```python
from build123d import *

# Parameters (mm, degrees)
SKETCH1_W                           = 170
SKETCH1_H                           = 60
SKETCH1_W_2                         = 53
SKETCH1_H_2                         = 30
BOSS_EXTRUDE1_DEPTH                 = 5
SKETCH3_W                           = 40
SKETCH3_H                           = 24
CUT_EXTRUDE1_DEPTH                  = 5
SKETCH5_R                           = 3
CUT_EXTRUDE2_DEPTH                  = 10
SKETCH6_R                           = 3
SKETCH6_R_2                         = 1.375
BOSS_EXTRUDE2_DEPTH                 = 5
SKETCH8_R                           = 2.375
SKETCH8_R_2                         = 1.375
BOSS_EXTRUDE3_DEPTH                 = 10
SKETCH9_W                           = 53
SKETCH9_H                           = 25
SKETCH9_W_2                         = 43
SKETCH9_H_2                         = 17.5
BOSS_EXTRUDE4_DEPTH                 = 5
SKETCH10_W                          = 3
SKETCH10_H                          = 17.5
SKETCH10_W_2                        = 5
SKETCH10_W_3                        = 2
BOSS_EXTRUDE5_DEPTH                 = 2
SKETCH11_W                          = 5
SKETCH11_H                          = 17.5
CUT_EXTRUDE5_DEPTH                  = 2
CHAMFER1_SIZE                       = 5
FILLET1_R                           = 5
SKETCH12_W                          = 43
SKETCH12_H                          = 32.847222222
SKETCH12_W_2                        = 60
SKETCH12_H_2                        = 24.8
CUT_EXTRUDE6_DEPTH                  = 105.522724802
FILLET2_R                           = 5
F_2_8_2_8_DIAMETER_HOLE1_AT_2_COUNT = 2
F_2_8_2_8_DIAMETER_HOLE1_AT_2_PITCH = 53.036757065
F_2_8_2_8_DIAMETER_HOLE1_AT_3_COUNT = 2
F_2_8_2_8_DIAMETER_HOLE1_AT_3_PITCH = 79.966896276
F_2_8_2_8_DIAMETER_HOLE1_AT_4_COUNT = 2
F_2_8_2_8_DIAMETER_HOLE1_AT_4_PITCH = 48.276707634
F_2_8_2_8_DIAMETER_HOLE1_AT_5_COUNT = 2
F_2_8_2_8_DIAMETER_HOLE1_AT_5_PITCH = 66.671976122
F_2_8_2_8_DIAMETER_HOLE1_AT_6_COUNT = 2
F_2_8_2_8_DIAMETER_HOLE1_AT_6_PITCH = 92.923433535
F_2_8_2_8_DIAMETER_HOLE1_AT_7_COUNT = 2
F_2_8_2_8_DIAMETER_HOLE1_AT_7_PITCH = 160.77550964
F_2_8_2_8_DIAMETER_HOLE1_AT_8_COUNT = 2
F_2_8_2_8_DIAMETER_HOLE1_AT_8_PITCH = 153.65124308


with BuildPart() as part:
    # Sketch1 → Boss-Extrude1 (new body)
    with BuildSketch(Plane(origin=(0, 0, 0), x_dir=(1, 0, 0), z_dir=(0, 1, 0))):
        Rectangle(SKETCH1_W, SKETCH1_H)
        with Locations((58.5, 45)):
            Rectangle(SKETCH1_W_2, SKETCH1_H_2)
    extrude(amount=BOSS_EXTRUDE1_DEPTH)

    # Sketch3 → Cut-Extrude1 (cut)
    with BuildSketch(Plane(origin=(0, 5, 0), x_dir=(1, 0, 0), z_dir=(0, 1, 0))):
        with Locations((12, 18)):
            Rectangle(SKETCH3_W, SKETCH3_H)
    extrude(amount=-CUT_EXTRUDE1_DEPTH, mode=Mode.SUBTRACT)

    # Sketch5 → Cut-Extrude2 (cut)
    with BuildSketch(Plane.XZ):
        with Locations(Location((-77.5, 22.5, 0), (0, 0, 270))):
            Circle(SKETCH5_R)
    extrude(amount=-CUT_EXTRUDE2_DEPTH, mode=Mode.SUBTRACT)

    # Sketch6 → Boss-Extrude2 (add)
    # profile 1 of 4: a face of its own
    with BuildSketch(Plane(origin=(0, 5, 0), x_dir=(1, 0, 0), z_dir=(0, 1, 0))):
        with Locations(Location((-71.03, -24.13, 0), (0, 0, 270))):
            Circle(SKETCH6_R)
        with Locations(Location((-71.03, -24.13, 0), (0, 0, 270))):
            Circle(SKETCH6_R_2, mode=Mode.SUBTRACT)
    # profile 2 of 4: a face of its own
    with BuildSketch(Plane(origin=(0, 5, 0), x_dir=(1, 0, 0), z_dir=(0, 1, 0))):
        with Locations(Location((-69.76, 24.13, 0), (0, 0, 270))):
            Circle(SKETCH6_R)
        with Locations(Location((-69.76, 24.13, 0), (0, 0, 270))):
            Circle(SKETCH6_R_2, mode=Mode.SUBTRACT)
    # profile 3 of 4: a face of its own
    with BuildSketch(Plane(origin=(0, 5, 0), x_dir=(1, 0, 0), z_dir=(0, 1, 0))):
        with Locations(Location((-18.96, -19.05, 0), (0, 0, 270))):
            Circle(SKETCH6_R)
        with Locations(Location((-18.96, -19.05, 0), (0, 0, 270))):
            Circle(SKETCH6_R_2, mode=Mode.SUBTRACT)
    # profile 4 of 4: a face of its own
    with BuildSketch(Plane(origin=(0, 5, 0), x_dir=(1, 0, 0), z_dir=(0, 1, 0))):
        with Locations(Location((-18.96, 8.89, 0), (0, 0, 270))):
            Circle(SKETCH6_R)
        with Locations(Location((-18.96, 8.89, 0), (0, 0, 270))):
            Circle(SKETCH6_R_2, mode=Mode.SUBTRACT)
    extrude(amount=BOSS_EXTRUDE2_DEPTH)

    # Sketch8 → Boss-Extrude3 (add)
    # profile 1 of 4: a face of its own
    with BuildSketch(Plane(origin=(0, 5, 0), x_dir=(1, 0, 0), z_dir=(0, 1, 0))):
        with Locations(Location((7.5, 3.5, 0), (0, 0, 270))):
            Circle(SKETCH8_R)
        with Locations(Location((7.5, 3.5, 0), (0, 0, 270))):
            Circle(SKETCH8_R_2, mode=Mode.SUBTRACT)
    # profile 2 of 4: a face of its own
    with BuildSketch(Plane(origin=(0, 5, 0), x_dir=(1, 0, 0), z_dir=(0, 1, 0))):
        with Locations(Location((7.5, -27.5, 0), (0, 0, 270))):
            Circle(SKETCH8_R)
        with Locations(Location((7.5, -27.5, 0), (0, 0, 270))):
            Circle(SKETCH8_R_2, mode=Mode.SUBTRACT)
    # profile 3 of 4: a face of its own
    with BuildSketch(Plane(origin=(0, 5, 0), x_dir=(1, 0, 0), z_dir=(0, 1, 0))):
        with Locations(Location((82.5, -27.5, 0), (0, 0, 270))):
            Circle(SKETCH8_R)
        with Locations(Location((82.5, -27.5, 0), (0, 0, 270))):
            Circle(SKETCH8_R_2, mode=Mode.SUBTRACT)
    # profile 4 of 4: a face of its own
    with BuildSketch(Plane(origin=(0, 5, 0), x_dir=(1, 0, 0), z_dir=(0, 1, 0))):
        with Locations(Location((82.5, 3.5, 0), (0, 0, 270))):
            Circle(SKETCH8_R)
        with Locations(Location((82.5, 3.5, 0), (0, 0, 270))):
            Circle(SKETCH8_R_2, mode=Mode.SUBTRACT)
    extrude(amount=BOSS_EXTRUDE3_DEPTH)

    # Sketch9 → Boss-Extrude4 (add)
    # profile 1 of 2: a face of its own
    with BuildSketch(Plane(origin=(0, 5, 0), x_dir=(1, 0, 0), z_dir=(0, 1, 0))):
        with Locations((58.5, 47.5)):
            Rectangle(SKETCH9_W, SKETCH9_H)
        with Locations((58.5, 46.25)):
            Rectangle(SKETCH9_W_2, SKETCH9_H_2, mode=Mode.SUBTRACT)
    # profile 2 of 2: a face of its own
    with BuildSketch(Plane(origin=(0, 5, 0), x_dir=(1, 0, 0), z_dir=(0, 1, 0))):
        with Locations((58.5, 20)):
            Rectangle(SKETCH9_W, SKETCH9_H)
        with Locations((58.5, 21.25)):
            Rectangle(SKETCH9_W_2, SKETCH9_H_2, mode=Mode.SUBTRACT)
    extrude(amount=BOSS_EXTRUDE4_DEPTH)

    # Sketch10 → Boss-Extrude5 (add)
    with BuildSketch(Plane(origin=(0, 5, 0), x_dir=(1, 0, 0), z_dir=(0, 1, 0))):
        with Locations((45.5, 21.25)):
            Rectangle(SKETCH10_W, SKETCH10_H)
        with Locations((59.5, 21.25)):
            Rectangle(SKETCH10_W_2, SKETCH10_H)
        with Locations((70, 21.25)):
            Rectangle(SKETCH10_W_3, SKETCH10_H)
        with Locations((45.5, 46.25)):
            Rectangle(SKETCH10_W, SKETCH10_H)
        with Locations((59.5, 46.25)):
            Rectangle(SKETCH10_W_2, SKETCH10_H)
        with Locations((70, 46.25)):
            Rectangle(SKETCH10_W_3, SKETCH10_H)
        with Locations((79, 21.25)):
            Rectangle(SKETCH10_W_3, SKETCH10_H)
        with Locations((79, 46.25)):
            Rectangle(SKETCH10_W_3, SKETCH10_H)
    extrude(amount=BOSS_EXTRUDE5_DEPTH)

    # Sketch11 → Cut-Extrude5 (cut)
    with BuildSketch(Plane(origin=(0, 10, 0), x_dir=(1, 0, 0), z_dir=(0, 1, 0))):
        with Locations((82.5, 21.25)):
            Rectangle(SKETCH11_W, SKETCH11_H)
        with Locations((82.5, 46.25)):
            Rectangle(SKETCH11_W, SKETCH11_H)
    extrude(amount=-CUT_EXTRUDE5_DEPTH, mode=Mode.SUBTRACT)

    # Chamfer1
    chamfer1_edges = [part.edges().sort_by_distance(p)[0] for p in [
        (-85, 2.5, 30),
        (-85, 2.5, -30),
        (-8, 2.5, -30),
        (32, 5, -60),
        (85, 5, -60),
    ]]
    chamfer(chamfer1_edges, length=CHAMFER1_SIZE)

    # Fillet1
    fillet1_edges = [part.edges().sort_by_distance(p)[0] for p in [
        (-8, 2.5, -6),
    ]]
    fillet(fillet1_edges, radius=FILLET1_R)

    # Sketch12 → Cut-Extrude6 (cut, through all)
    with BuildSketch(Plane(origin=(0, 5, 0), x_dir=(1, 0, 0), z_dir=(0, 1, 0))):
        with Locations((-46.5, 0)):
            Rectangle(SKETCH12_W, SKETCH12_H)
        with Locations((45, -12)):
            Rectangle(SKETCH12_W_2, SKETCH12_H_2)
    extrude(amount=-CUT_EXTRUDE6_DEPTH, mode=Mode.SUBTRACT)

    # Fillet2
    fillet2_edges = [part.edges().sort_by_distance(p)[0] for p in [
        (-25, 2.5, -16.423611111),
        (-25, 2.5, 16.423611111),
        (-68, 2.5, 16.423611111),
        (-68, 2.5, -16.423611111),
        (75, 2.5, -0.4),
        (75, 2.5, 24.4),
        (15, 2.5, 24.4),
        (15, 2.5, -0.4),
    ]]
    fillet(fillet2_edges, radius=FILLET2_R)

    # Sketch14 → Ø2.8 (2.8) Diameter Hole1 (revolve, cut)
    with BuildSketch(Plane(origin=(-69.76, 5, -24.13), x_dir=(0, 0, 1), z_dir=(1, 0, 0))):
        Polygon((0, 0), (0, 10.841204867), (1.4, 10), (1.4, 0), align=None)
    f_2_8_2_8_diameter_hole1 = revolve(axis=Axis((-69.76, 11.35, -24.13), (0, -1, 0)), mode=Mode.SUBTRACT)

    # Ø2.8 (2.8) Diameter Hole1 at 2: Ø2.8 (2.8) Diameter Hole1 ×2
    with Locations(*[Vector(0.9578262852211514, 0, 0.2873478855663455) * (i * F_2_8_2_8_DIAMETER_HOLE1_AT_2_PITCH) for i in range(1, F_2_8_2_8_DIAMETER_HOLE1_AT_2_COUNT)]):
        add(f_2_8_2_8_diameter_hole1, mode=Mode.SUBTRACT)

    # Ø2.8 (2.8) Diameter Hole1 at 3: Ø2.8 (2.8) Diameter Hole1 ×2
    with Locations(*[Vector(0.9661497894509072, 0, 0.2579817519592574) * (i * F_2_8_2_8_DIAMETER_HOLE1_AT_3_PITCH) for i in range(1, F_2_8_2_8_DIAMETER_HOLE1_AT_3_COUNT)]):
        add(f_2_8_2_8_diameter_hole1, mode=Mode.SUBTRACT)

    # Ø2.8 (2.8) Diameter Hole1 at 4: Ø2.8 (2.8) Diameter Hole1 ×2
    with Locations(*[Vector(-0.02630668208823303, 0, 0.9996539193528472) * (i * F_2_8_2_8_DIAMETER_HOLE1_AT_4_PITCH) for i in range(1, F_2_8_2_8_DIAMETER_HOLE1_AT_4_COUNT)]):
        add(f_2_8_2_8_diameter_hole1, mode=Mode.SUBTRACT)

    # Ø2.8 (2.8) Diameter Hole1 at 5: Ø2.8 (2.8) Diameter Hole1 ×2
    with Locations(*[Vector(0.7619393177594593, 0, 0.6476484200955406) * (i * F_2_8_2_8_DIAMETER_HOLE1_AT_5_PITCH) for i in range(1, F_2_8_2_8_DIAMETER_HOLE1_AT_5_COUNT)]):
        add(f_2_8_2_8_diameter_hole1, mode=Mode.SUBTRACT)

    # Ø2.8 (2.8) Diameter Hole1 at 6: Ø2.8 (2.8) Diameter Hole1 ×2
    with Locations(*[Vector(0.8314372065320044, 0, 0.5556187286208567) * (i * F_2_8_2_8_DIAMETER_HOLE1_AT_6_PITCH) for i in range(1, F_2_8_2_8_DIAMETER_HOLE1_AT_6_COUNT)]):
        add(f_2_8_2_8_diameter_hole1, mode=Mode.SUBTRACT)

    # Ø2.8 (2.8) Diameter Hole1 at 7: Ø2.8 (2.8) Diameter Hole1 ×2
    with Locations(*[Vector(0.9470347837238248, 0, 0.3211309988418566) * (i * F_2_8_2_8_DIAMETER_HOLE1_AT_7_PITCH) for i in range(1, F_2_8_2_8_DIAMETER_HOLE1_AT_7_COUNT)]):
        add(f_2_8_2_8_diameter_hole1, mode=Mode.SUBTRACT)

    # Ø2.8 (2.8) Diameter Hole1 at 8: Ø2.8 (2.8) Diameter Hole1 ×2
    with Locations(*[Vector(0.99094544858852, 0, 0.13426510314187035) * (i * F_2_8_2_8_DIAMETER_HOLE1_AT_8_PITCH) for i in range(1, F_2_8_2_8_DIAMETER_HOLE1_AT_8_COUNT)]):
        add(f_2_8_2_8_diameter_hole1, mode=Mode.SUBTRACT)


solid = part.part
```
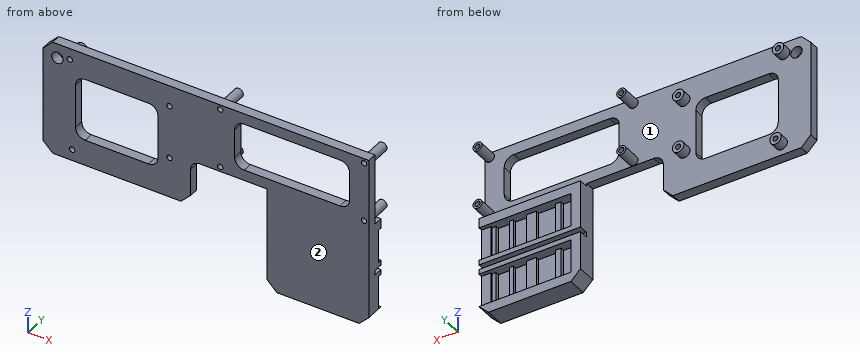
Geometry: final body of the model. Coordinates: model frame, mm. Face numbers are marked on the shaded views. Round coordinates to 2 decimals unless told otherwise and drop trailing zeros. Write each loop counter-clockwise with the first axis right and the second up, starting at its lowest first coordinate (ties: lowest second). Pieces come first, ordered by that corner, then holes.
Item 1: Section query A-A (z = 8). Return loops of the section in (x, y).
Item 2: Section query D-D (y = 2.5). Give the number of separate pieces and of enclosed holes in the cut face, plus the area to 3 significant figures.
Item 3: Pin query (flat end, axial travel): P1, Ø6, axis at x = -55.5, z = -15.5, coming from the +Y side; P2, Ø1, axis at x = -58, y = 4.5, coming from the -Z side; P3, Ø4, axis at x = 60, z = -49, coming from the +Y side. Return the tip coordinate at first contact, or that it passes through.
Item 4: Material intervals for L1, parallel to X at y = 2.05, z = -3.5; L2, parallel to X at y = 5.75, z = -28; L3, parallel to X at y = 2.85, z = -24.13, sorted ascending.
Item 5: Section query C-C (z = -48). Return loops of the section in (x, y).
Item 6: Section query B-B (x = -77.5). Return loops of the section in (y, z).
Item 7: Mould query, pull axis X, two halves, no side actions, for the marked faces 1 and 2. Classes: +X half, -X half, draft (parallel to the pull), parting line (faces both ways), or undercut.
Completed:
1. outline: (-85, 0) - (-68, 0) - (-68, 5) - (-85, 5) - close; (-25, 0) - (15, 0) - (15, 5) - (-25, 5) - close; (75, 0) - (85, 0) - (85, 5) - (75, 5) - close
2. separate pieces: 1
2. enclosed holes: 11
2. area: 7,840 mm2
3. P1: stops at y = 5
3. P2: stops at z = -30
3. P3: stops at y = 7
4. L1: x = -85 to -68, -25 to 6.1, 8.9 to 81.1, 83.9 to 85
4. L2: x = 32 to 37, 44 to 47, 57 to 62, 69 to 71, 78 to 85
4. L3: x = -85 to -71.16, -68.36 to -8, 32 to 85
5. outline: (32, 0) - (85, 0) - (85, 8) - (80, 8) - (80, 7) - (78, 7) - (78, 5) - (71, 5) - (71, 7) - (69, 7) - (69, 5) - (62, 5) - (62, 7) - (57, 7) - (57, 5) - (47, 5) - (47, 7) - (44, 7) - (44, 5) - (37, 5) - (37, 10) - (32, 10) - close
6. outline: (0, -30) - (5, -30) - (5, 19.5) - (0, 19.5) - close; (0, 25.5) - (5, 25.5) - (5, 30) - (0, 30) - close
7. face 1: undercut
7. face 2: draft
